Input: part model. Units: mm. Frame: model coordinates. Face numbers are marked on the shaded views. A direction names the side the tool comes from. Give positions to 0.01 mm unless a question says otherwise; leave off trailing zeros. Write each loop counter-clockwise with the first axis right and the second up, starting at its lowest first coordinate (ties: lowest second). Pieces come first, ordered by that corner, then holes. Notation, with made-up numbers: (80.25, 70) - (98.25, 70) arc R29 cw to (98.25, 100) - close; hole circle Ø7 at (-23, -19). An arc over 180 degrees is marked (long way). Answer as CSV lines item,"result".
```python
from build123d import *

# Parameters (mm, degrees)
BOSS_EXTRUDE1_DEPTH = 10.181166667
SKETCH2_R           = 5
CUT_EXTRUDE1_DEPTH  = 1
CUT_EXTRUDE2_DEPTH  = 7.5


with BuildPart() as part:
    # Sketch1 → Boss-Extrude1 (new body)
    with BuildSketch(Plane.XY):
        with BuildLine():
            Line((-6.59848134, 3.41844841), (-6.587531167, 3.487972592))
            ThreePointArc((-6.587531167, 3.487972592), (-5.270745663, 5.270745663), (-3.487972592, 6.587531167))
            Line((-3.487972592, 6.587531167), (-3.41844841, 6.59848134))
            ThreePointArc((-3.41844841, 6.59848134), (-3.64449132, 9.108619705), (-3.367456173, 11.613642965))
            ThreePointArc((-3.367456173, 11.613642965), (8.550335198, 8.550335198), (11.613642965, -3.367456173))
            ThreePointArc((11.613642965, -3.367456173), (9.108619705, -3.64449132), (6.59848134, -3.41844841))
            Line((6.59848134, -3.41844841), (6.587531167, -3.487972592))
            ThreePointArc((6.587531167, -3.487972592), (5.270745663, -5.270745663), (3.487972592, -6.587531167))
            Line((3.487972592, -6.587531167), (3.41844841, -6.59848134))
            ThreePointArc((3.41844841, -6.59848134), (3.64449132, -9.108619705), (3.367456173, -11.613642965))
            ThreePointArc((3.367456173, -11.613642965), (-8.550335198, -8.550335198), (-11.613642965, 3.367456173))
            ThreePointArc((-11.613642965, 3.367456173), (-9.108619705, 3.64449132), (-6.59848134, 3.41844841))
        make_face()
    extrude(amount=BOSS_EXTRUDE1_DEPTH)

    # Sketch2 → Cut-Extrude1 (cut)
    with BuildSketch(Plane(origin=(0, 0, 0), x_dir=(-1, 0, 0), z_dir=(0, 0, -1))):
        Circle(SKETCH2_R)
    extrude(amount=-CUT_EXTRUDE1_DEPTH, mode=Mode.SUBTRACT)

    # Sketch3 → Cut-Extrude2 (cut)
    with BuildSketch(Plane.XY.offset(10.181166667)):
        with BuildLine():
            Line((9.15948917, 2.425242905), (9.281504474, 2.548391591))
            ThreePointArc((9.281504474, 2.548391591), (6.805902769, 6.805902769), (2.548391591, 9.281504474))
            Line((2.548391591, 9.281504474), (2.425242905, 9.15948917))
            ThreePointArc((2.425242905, 9.15948917), (2.740607895, 6.73570708), (2.425506361, 4.311890725))
            Line((2.425506361, 4.311890725), (2.4714668, 4.200130912))
            ThreePointArc((2.4714668, 4.200130912), (3.445957619, 3.445957619), (4.200130912, 2.4714668))
            Line((4.200130912, 2.4714668), (4.238745161, 2.405843866))
            ThreePointArc((4.238745161, 2.405843866), (6.481209779, 2.737203521), (8.738209013, 2.5264875))
            ThreePointArc((8.738209013, 2.5264875), (8.949427835, 2.478273365), (9.15948917, 2.425242905))
        make_face()
    cut_extrude2 = extrude(amount=-CUT_EXTRUDE2_DEPTH, mode=Mode.SUBTRACT)

    # Mirror1: Cut-Extrude2 across plane
    add(cut_extrude2.mirror(Plane(origin=(0, 0, 0), x_dir=(0, 0, 1), z_dir=(0.7071067811865475, 0.7071067811865477, 0))), mode=Mode.SUBTRACT)


solid = part.part
```
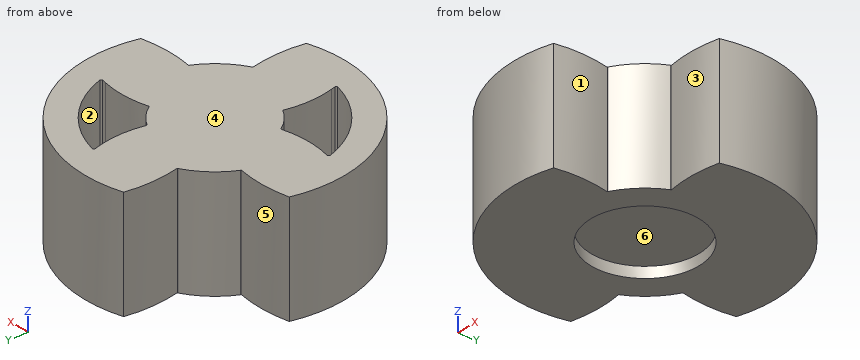
Item 1: Cut plane D-D on z = 2. Return the cut outline in (x, y).
The answers:
outline,"(-11.61, 3.37) arc R12.09 ccw to (3.37, -11.61) arc R12.63 ccw to (3.42, -6.6) - (3.49, -6.59) arc R7.45 ccw to (6.59, -3.49) - (6.6, -3.42) arc R12.63 ccw to (11.61, -3.37) arc R12.09 ccw to (-3.37, 11.61) arc R12.63 ccw to (-3.42, 6.6) - (-3.49, 6.59) arc R7.45 ccw to (-6.59, 3.49) - (-6.6, 3.42) arc R12.63 ccw to start"
Item 2: Cut plane A-A on y = 0. Return the cut outline in (x, z), plus the area to 3 significant figures.
The answers:
outline,"(-12.09, 0) - (-5, 0) - (-5, 1) - (5, 1) - (5, 0) - (12.09, 0) - (12.09, 10.18) - (-12.09, 10.18) - close"
area,"236 mm²"
Item 3: Mould query, pull axis Y, two halves, no side actions, for the marked faces 3, 4, 5 and 6. Classes: +Y half, -Y half, draft (parallel to the pull), parting line (faces both ways), or undercut.
The answers:
face 3,"-Y half"
face 4,"draft"
face 5,"+Y half"
face 6,"undercut"
Item 4: Cut plane B-B on z = 0.5. Return the cut outline in (x, y).
The answers:
outline,"(-11.61, 3.37) arc R12.09 ccw to (3.37, -11.61) arc R12.63 ccw to (3.42, -6.6) - (3.49, -6.59) arc R7.45 ccw to (6.59, -3.49) - (6.6, -3.42) arc R12.63 ccw to (11.61, -3.37) arc R12.09 ccw to (-3.37, 11.61) arc R12.63 ccw to (-3.42, 6.6) - (-3.49, 6.59) arc R7.45 ccw to (-6.59, 3.49) - (-6.6, 3.42) arc R12.63 ccw to start; hole circle Ø10 at (0, 0)"
Item 5: Reachability of the marked faces 1 and 2 from +Z, -Z, +X, -X, +Y, -Y: full face, straight path, thin tool, end or side. Return the list, or none.
The answers:
face 1,"+Z, -Z, +X"
face 2,"+Z"
Item 6: Ray query, line 1 (Y direction, x = 0, z = 0.45); line 2 (Z direction, x = 2.5, y = -3.5); line 3 (X direction, y = 8.5, z = 7.75). Return the intervals inside material, ascending. Write a range as from..to.
The answers:
line 1,"-12.09..-5, 5..12.09"
line 2,"1..10.18"
line 3,"-3.64..2.57, 4.52..8.6"
Item 7: Contact query for flat-ended pins moving along their axis: pin 1 (1 mm diameter, centred on y = 5, z = 8, fed in from -X); pin 2 (1.5 mm diameter, centred on y = -4, z = 6, fed in from +X); pin 3 (2 mm diameter, centred on y = 9, z = 3.5, fed in from +X). Output: stop coordinate, or through.
The answers:
pin 1,"x = -5.94"
pin 2,"x = 11.65"
pin 3,"x = 9.07"
